The model under review builds one solid part; all positions refer to its coordinate system, in mm. Face numbers are marked on the shaded views. A direction names the side the tool comes from. Give positions to 0.01 mm unless a question says otherwise; leave off trailing zeros. Loops run counter-clockwise (first coordinate to the right, second up) from the corner with the lowest first, then second, coordinate; pieces in that order, holes last. Notation, with made-up numbers: M 48.5,-25 L 66.5,-25 A18 ccw 66.5,5 Z; hole C 24,2 d1. An arc over 180 degrees is marked long. Return JSON: item names as keys, results as strings.
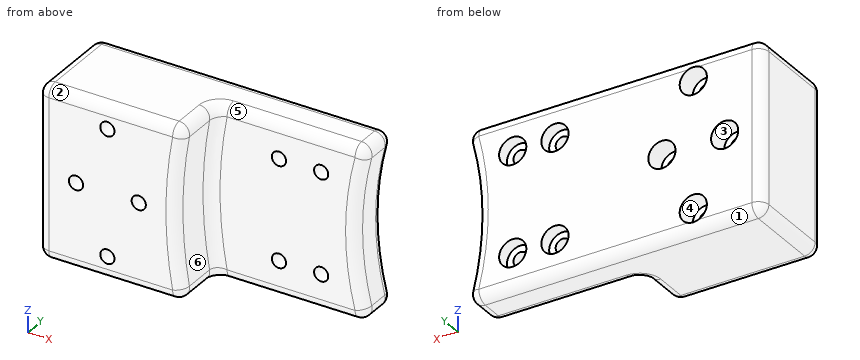
```python
from build123d import *

# Parameters (mm, degrees)
BOSS_EXTRUDE1_DEPTH            = 20.5
SKETCH2_R                      = 70
CUT_EXTRUDE1_DEPTH             = 41
SKETCH3_R                      = 100
CUT_EXTRUDE2_DEPTH             = 41
FILLET1_R                      = 2.5
CBORE_FOR_M3_SHCS1_D           = 3.4
CBORE_FOR_M3_SHCS1_DEPTH       = 45
CBORE_FOR_M3_SHCS1_CBORE_D     = 6.5
CBORE_FOR_M3_SHCS1_CBORE_DEPTH = 5
CBORE_FOR_M3_SHCS1_TIP         = 1.021463052
CBORE_FOR_M3_SHCS2_D           = 3.4
CBORE_FOR_M3_SHCS2_DEPTH       = 45
CBORE_FOR_M3_SHCS2_CBORE_D     = 6.5
CBORE_FOR_M3_SHCS2_CBORE_DEPTH = 3
CBORE_FOR_M3_SHCS2_TIP         = 1.021463052


with BuildPart() as part:
    # Sketch1 → Boss-Extrude1 (new body, symmetric)
    with BuildSketch(Plane.XY):
        Polygon((-70, 0), (-105, 0), (-105, -12.7), (-143, -12.7), (-143, 10), (-70, 10), align=None)
    extrude(amount=BOSS_EXTRUDE1_DEPTH, both=True)

    # Sketch2 → Cut-Extrude1 (cut)
    with BuildSketch(Plane(origin=(0, 10, 0), x_dir=(1, 0, 0), z_dir=(0, 1, 0))):
        with Locations((-5, 0)):
            Circle(SKETCH2_R)
    extrude(amount=-CUT_EXTRUDE1_DEPTH, mode=Mode.SUBTRACT)

    # Sketch3 → Cut-Extrude2 (cut)
    with BuildSketch(Plane(origin=(0, 0, 0), x_dir=(1, 0, 0), z_dir=(0, 1, 0))):
        with Locations((-10, 0)):
            Circle(SKETCH3_R)
    extrude(amount=-CUT_EXTRUDE2_DEPTH, mode=Mode.SUBTRACT)

    # Fillet1
    fillet1_edges = [part.edges().sort_by_distance(p)[0] for p in [
        (-143, -12.7, 0),
        (-143, 10, 0),
        (-143, -1.35, 20.5),
        (-125.438098655, -12.7, 20.5),
        (-107.465467276, 10, -20.5),
        (-71.930934552, 5, -20.5),
        (-107.465467276, 10, 20.5),
        (-75, 0, 0),
        (-71.930934552, 5, 20.5),
        (-75, 10, 0),
        (-89.903565931, 0, 20.5),
        (-107.876197311, -6.35, -20.5),
        (-110, -12.7, 0),
        (-107.876197311, -6.35, 20.5),
        (-110, 0, 0),
        (-89.903565931, 0, -20.5),
        (-125.438098655, -12.7, -20.5),
        (-143, -1.35, -20.5),
    ]]
    fillet(fillet1_edges, radius=FILLET1_R)

    # CBORE for M3 SHCS1
    with Locations(Plane(origin=(0, 10, 0), x_dir=(1, 0, 0), z_dir=(0, 1, 0))):
        with Locations((-134, 0), (-119, 0), (-126.5, 15), (-126.5, -15)):
            CounterBoreHole(CBORE_FOR_M3_SHCS1_D / 2, CBORE_FOR_M3_SHCS1_CBORE_D / 2, CBORE_FOR_M3_SHCS1_CBORE_DEPTH, depth=CBORE_FOR_M3_SHCS1_DEPTH)
            with Locations((0, 0, -(CBORE_FOR_M3_SHCS1_DEPTH + CBORE_FOR_M3_SHCS1_TIP / 2))):  # 118° drill point
                Cone(0, CBORE_FOR_M3_SHCS1_D / 2, CBORE_FOR_M3_SHCS1_TIP, mode=Mode.SUBTRACT)

    # CBORE for M3 SHCS2
    with Locations(Plane(origin=(0, 10, 0), x_dir=(1, 0, 0), z_dir=(0, 1, 0))):
        with Locations((-93.432542511, 12), (-93.432542511, -12), (-83.340506358, 12), (-83.340506358, -12)):
            CounterBoreHole(CBORE_FOR_M3_SHCS2_D / 2, CBORE_FOR_M3_SHCS2_CBORE_D / 2, CBORE_FOR_M3_SHCS2_CBORE_DEPTH, depth=CBORE_FOR_M3_SHCS2_DEPTH)
            with Locations((0, 0, -(CBORE_FOR_M3_SHCS2_DEPTH + CBORE_FOR_M3_SHCS2_TIP / 2))):  # 118° drill point
                Cone(0, CBORE_FOR_M3_SHCS2_D / 2, CBORE_FOR_M3_SHCS2_TIP, mode=Mode.SUBTRACT)


solid = part.part
```
1) Consider section D-D on y = -8.5. Write out the cut boundary in (x, z), then the cut area to 3 significant figures.
From the geometry:
{"outline": "M -143,-18 A2.5 ccw -140.5,-20.5 L -110.91,-20.5 A2.5 ccw -108.45,-17.56 A100 cw -108.45,17.56 A2.5 ccw -110.91,20.5 L -140.5,20.5 A2.5 ccw -143,18 Z; hole C -134,0 d3.4; hole C -126.5,-15 d3.4; hole C -126.5,15 d3.4; hole C -119,0 d3.4", "area": "1,340 mm²"}
2) The part is to be moulded in two halves that separate along Z. For the marked faces 1, 2 and 3, say which applies: released by +Z, released by -Z, zero draft, split by the parting line, or undercut.
From the geometry:
{"face 1": "released by -Z", "face 2": "released by +Z", "face 3": "undercut"}
3) Tool access review of the marked faces 4, 5 and 6: name each direction out of +Z, -Z, +X, -X, +Y, -Y from which nothing blocks a thin tool from reaching the whole face with its end or side.
From the geometry:
{"face 4": "+Y", "face 5": "+Z, +X, -Y", "face 6": "+X, -Y"}
4) Consider section A-A on z = 0. Write out the cut boundary in (x, y), then the cut area to 3 significant figures.
From the geometry:
{"outline": "M -143,-10.2 A2.5 ccw -140.5,-12.7 L -135.7,-12.7 L -135.7,5 L -137.25,5 L -137.25,10 L -140.5,10 A2.5 ccw -143,7.5 Z; M -132.3,-12.7 L -120.7,-12.7 L -120.7,5 L -122.25,5 L -122.25,10 L -130.75,10 L -130.75,5 L -132.3,5 Z; M -117.3,-12.7 L -112.5,-12.7 A2.5 ccw -110,-10.2 L -110,-2.5 A2.5 cw -107.5,0 L -77.5,0 A2.5 ccw -75,2.5 L -75,7.5 A2.5 ccw -77.5,10 L -115.75,10 L -115.75,5 L -117.3,5 Z", "area": "908 mm²"}
5) Insertion check: pin 1 (1.5 mm diameter, centred on x = -84, z = -4, fed in from -Y); pin 2 (2 mm diameter, centred on x = -134, z = 0, fed in from -Y); pin 3 (4 mm diameter, centred on x = -93.43, z = 12, fed in from +Y); pin 4 (2 mm diameter, centred on x = -126.5, z = -16, fed in from +Y). Each pin has a flat end and moves straight along its axis. Give the tip position at first contact, or say it passes through.
From the geometry:
{"pin 1": "y = 0", "pin 2": "through", "pin 3": "y = 7", "pin 4": "y = 5"}
6) Wall thickness on L1, parallel to Z at x = -134, y = 0.5; L2, parallel to Z at x = -126.5, y = -6.5; L3, parallel to Y at x = -101, z = 14.5: over which ranges is each line inside the solid? List them lowest first. Write a range as from..to.
From the geometry:
{"L1": "-20.5..-1.7, 1.7..20.5", "L2": "-20.5..-16.7, -13.3..13.3, 16.7..20.5", "L3": "0..10"}
7) Consider section C-C on x = -126.5. Write out the cut boundary in (y, z).
From the geometry:
{"outline": "M -12.7,-18 A2.5 ccw -10.2,-20.5 L 7.5,-20.5 A2.5 ccw 9.99,-18.25 L 5,-18.25 L 5,-16.7 L -12.7,-16.7 Z; M -12.7,-13.3 L 5,-13.3 L 5,-11.75 L 10,-11.75 L 10,11.75 L 5,11.75 L 5,13.3 L -12.7,13.3 Z; M -12.7,16.7 L 5,16.7 L 5,18.25 L 9.99,18.25 A2.5 ccw 7.5,20.5 L -10.2,20.5 A2.5 ccw -12.7,18 Z"}
8) Consider section B-B on x = -119. Write out the cut boundary in (y, z), then the cut area to 3 significant figures.
From the geometry:
{"outline": "M -12.7,-18 A2.5 ccw -10.2,-20.5 L 7.5,-20.5 A2.5 ccw 10,-18 L 10,-3.25 L 5,-3.25 L 5,-1.7 L -12.7,-1.7 Z; M -12.7,1.7 L 5,1.7 L 5,3.25 L 10,3.25 L 10,18 A2.5 ccw 7.5,20.5 L -10.2,20.5 A2.5 ccw -12.7,18 Z", "area": "833 mm²"}
